Input: part model. Units: mm. Frame: model coordinates. Face numbers are marked on the shaded views. Round coordinates to 2 decimals unless told otherwise and drop trailing zeros. Order: outer loops, then holes, each group sorted by start corner. A loop starts at its lowest first (then second) coordinate and runs counter-clockwise, first axis right, second up. Notation, with made-up numbers: (70, 15.5) -> (121, 15.5) arc R18 ccw to (121, 43.5) -> close; hole circle Ø1 at (47, 10). An arc over 180 degrees is marked (long way). Answer as CSV lines item,"result". Start each with the question number.
1) Section query A-A, the plane y = 0. Output: boundary loops of the cut face in (x, z), and give its area (3 significant figures).
2) First-contact query: P1, Ø1, axis at x = 1, y = -6, coming from the +Z side; P2, Ø6.5, axis at x = -0.5, y = 1.5, coming from the +Z side; P3, Ø4, axis at y = -8, z = 3.5, coming from the +X side. Flat tips, straight axial feed; report the tip coordinate or a pass-through.
3) Section query C-C, the plane z = 6. Output: boundary loops of the cut face in (x, y).
4) Mould query, pull axis Y, two halves, no side actions, for the marked faces 1, 2 and 3. Classes: +Y half, -Y half, draft (parallel to the pull), parting line (faces both ways), or undercut.
5) Line query: L1, parallel to Y at x = 0, z = 10; L2, parallel to Z at x = -1.5, y = -0.5. Output: solid intervals per line, ascending.
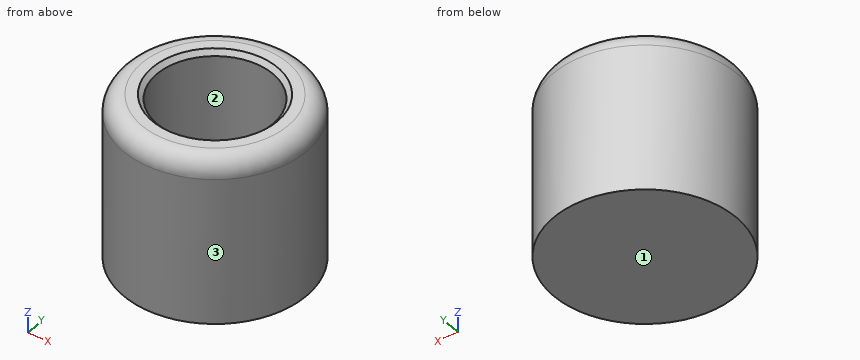
Autodesk Fusion 360 part; units mm, degrees
sketch "Sketch1" plane through (0, 0, 0) normal (0, 1, 0) x (1, 0, 0)
  line L0 (0, 0) -> (10, 0)
  line L1 (10, 0) -> (10, -3)
  line L2 (10, -3) -> (0, -3)
  line L3 (0, -3) -> (0, 0)
  line L4 (0, -3) -> (6.35, -3)
  line L5 (10, -3) -> (6.35, -3)
  line L6 (6.35, -3) -> (10, -3)
  line L7 (10, -3) -> (10, -18)
  line L8 (10, -18) -> (6.35, -18)
  line L9 (6.35, -18) -> (6.35, -3)
  dimension "d1" = 10
  dimension "d2" = 3
  dimension "d3" = 6.35
  dimension "d5" = 15
revolve "Revolve1" add sketch "Sketch1" angle 360 about axis through (0, 0, 3) along (0, 0, -1)
fillet "Fillet1" radius 2 1 edges at (-9.3233, -3.6162, 18)
chamfer "Chamfer1" distance 0.5 angle 45 1 edges at (-5.9203, -2.2963, 18)
Findings:
1,outline,"(-10, 0) -> (10, 0) -> (10, 16) arc R2 ccw to (8, 18) -> (6.85, 18) -> (6.35, 17.5) -> (6.35, 3) -> (-6.35, 3) -> (-6.35, 17.5) -> (-6.85, 18) -> (-8, 18) arc R2 ccw to (-10, 16) -> close"
1,area,"168 mm^2"
2,P1,"stops at z = 17.73"
2,P2,"stops at z = 3"
2,P3,"stops at x = 8"
3,outline,"circle Ø20 at (0, 0); hole circle Ø12.7 at (0, 0)"
4,face 1,"draft"
4,face 2,"undercut"
4,face 3,"parting line"
5,L1,"y = -10 to -6.35, 6.35 to 10"
5,L2,"z = 0 to 3"
